from build123d import *

# Parameters (mm, degrees)
SKETCH2_R           = 1.5
BOSS_EXTRUDE2_DEPTH = 3


with BuildPart() as part:
    # Sketch2 → Boss-Extrude2 (new body)
    with BuildSketch(Plane.XY):
        with BuildLine():
            Line((33.856406461, -4.911436862), (20, -2.911436862))
            Line((20, -2.911436862), (8.072676136, 9.818872958))
            ThreePointArc((8.072676136, 9.818872958), (-5.173839679, 11.745880003), (-12.077884766, 0.277763382))
            ThreePointArc((-12.077884766, 0.277763382), (-13.37688471, -0.097129684), (-14.542044827, -0.782948586))
            ThreePointArc((-14.542044827, -0.782948586), (-14.504838322, -1.090725234), (-14.461118588, -1.3976444))
            ThreePointArc((-14.461118588, -1.3976444), (-13.158157346, -1.758528961), (-11.806390286, -1.78444193))
            ThreePointArc((-11.806390286, -1.78444193), (-11.67804324, -2.310249297), (-11.526291359, -2.829785359))
            ThreePointArc((-11.526291359, -2.829785359), (-12.683999488, -3.528110178), (-13.631954743, -4.492125996))
            ThreePointArc((-13.631954743, -4.492125996), (-13.516357561, -4.779785658), (-13.394691015, -5.064931306))
            ThreePointArc((-13.394691015, -5.064931306), (-12.042723303, -5.076287839), (-10.73030982, -4.751454786))
            ThreePointArc((-10.73030982, -4.751454786), (-10.470247132, -5.226127042), (-10.189200244, -5.688684064))
            ThreePointArc((-10.189200244, -5.688684064), (-11.126720661, -6.662850955), (-11.792869471, -7.839367605))
            ThreePointArc((-11.792869471, -7.839367605), (-11.606759368, -8.087306749), (-11.415437385, -8.331246676))
            ThreePointArc((-11.415437385, -8.331246676), (-10.106597569, -7.992301252), (-8.922976471, -7.338859012))
            ThreePointArc((-8.922976471, -7.338859012), (-8.548920985, -7.730048027), (-8.15773197, -8.104103513))
            ThreePointArc((-8.15773197, -8.104103513), (-8.81117421, -9.287724611), (-9.150119633, -10.596564427))
            ThreePointArc((-9.150119633, -10.596564427), (-8.906179706, -10.787886411), (-8.658240563, -10.973996513))
            ThreePointArc((-8.658240563, -10.973996513), (-7.481723913, -10.307847704), (-6.507557022, -9.370327286))
            ThreePointArc((-6.507557022, -9.370327286), (-6.045, -9.651374174), (-5.570327744, -9.911436862))
            ThreePointArc((-5.570327744, -9.911436862), (-5.895160797, -11.223850345), (-5.883804264, -12.575818057))
            ThreePointArc((-5.883804264, -12.575818057), (-5.598658616, -12.697484603), (-5.310998954, -12.813081785))
            ThreePointArc((-5.310998954, -12.813081785), (-4.346983136, -11.86512653), (-3.648658316, -10.707418401))
            ThreePointArc((-3.648658316, -10.707418401), (-3.129122255, -10.859170282), (-2.603314888, -10.987517329))
            ThreePointArc((-2.603314888, -10.987517329), (-2.577401919, -12.339284388), (-2.216517358, -13.64224563))
            ThreePointArc((-2.216517358, -13.64224563), (-1.909598192, -13.685965364), (-1.601821544, -13.723171869))
            ThreePointArc((-1.601821544, -13.723171869), (-0.916002642, -12.558011752), (-0.541109576, -11.259011808))
            ThreePointArc((-0.541109576, -11.259011808), (0, -11.271127042), (0.541109576, -11.259011808))
            ThreePointArc((0.541109576, -11.259011808), (0.916002642, -12.558011752), (1.601821544, -13.723171869))
            ThreePointArc((1.601821544, -13.723171869), (1.909598192, -13.685965364), (2.216517358, -13.64224563))
            ThreePointArc((2.216517358, -13.64224563), (2.577401919, -12.339284388), (2.603314888, -10.987517329))
            ThreePointArc((2.603314888, -10.987517329), (3.129122255, -10.859170282), (3.648658316, -10.707418401))
            ThreePointArc((3.648658316, -10.707418401), (4.346983136, -11.86512653), (5.310998954, -12.813081785))
            ThreePointArc((5.310998954, -12.813081785), (5.598658616, -12.697484603), (5.883804264, -12.575818057))
            ThreePointArc((5.883804264, -12.575818057), (5.895160797, -11.223850345), (5.570327744, -9.911436862))
            ThreePointArc((5.570327744, -9.911436862), (6.876145849, -9.125307162), (8.072676136, -8.181127042))
            Line((8.072676136, -8.181127042), (16, -11.911436862))
            Line((16, -11.911436862), (36, -11.911436862))
            Line((36, -11.911436862), (40, -13.911436862))
            ThreePointArc((40, -13.911436862), (43.70240259, -12.65581862), (42.40824957, -8.966708962))
            Line((42.40824957, -8.966708962), (33.856406461, -4.911436862))
        make_face()
        with Locations((41.229904242, -11.451628378)):
            Circle(SKETCH2_R, mode=Mode.SUBTRACT)
        with Locations((0, 0.818872958)):
            Circle(SKETCH2_R, mode=Mode.SUBTRACT)
    extrude(amount=BOSS_EXTRUDE2_DEPTH)


solid = part.part
Work out the finished part from the listing and answer in its coordinate system (mm). A direction names the side the tool comes from. Give positions to 0.01 mm unless a question says otherwise; leave off trailing zeros. Loops run counter-clockwise (first coordinate to the right, second up) from the corner with the lowest first, then second, coordinate; pieces in that order, holes last. Notation, with made-up numbers: (-3, 15.5) -> (38, 15.5) arc R20 ccw to (38, 19.5) -> close; hole circle Ø7 at (88.25, 1). An arc over 180 degrees is marked (long way). Use a Markdown table: item, result. Add a question column.
1. Section C-C on x = 38 is taken. Determine the outline of the cut face in (y, z), and give its area (3 significant figures).
2. A flat-ended cylindrical pin translates along its axis: pin 1 Ø2.5 at (x, y) = (0, 0.82) entering from +Z. Find the tip coordinate at first contact, or state that the pin passes through.
3. Section D-D on y = 3.75 is taken. Determine the outline of the cut face in (x, z), and give its area (3 significant figures).
4. Find the intervals of material crossed by probe 1 along Y at (x, z) = (0, 2.1); probe 2 along X at (y, z) = (-10.5, 0.95); probe 3 along X at (y, z) = (-12, 2.6), in increasing order.
5. Section A-A on x = 0 is taken. Determine the outline of the cut face in (y, z).
6. Section B-B on z = 2.4 is taken. State how many separate pieces and enclosed holes the cut face has, and give its area (3 significant figures).
7. Determine the mould class of faces 4 (the flat face through (8, -3, 0)), 5 (the cylindrical face through (-4.99, 11.83, 1.48)), 6 (the cylindrical face through (-4.36, -11.88, 1.48)) for opening direction X: released by +X, released by -X, zero draft, split by the parting line, or undercut.
8. For faces 1 (the cylindrical face through (-0.01, -11.27, 1.48)), 2 (the cylindrical face through (2.575, -12.358, 1.479)), 3 (the flat face through (38.192, -6.967, 1.479)), determine the directions among +Z, -Z, +X, -X, +Y, -Y from which every point of the face is accessible in a straight line to the end or side of a thin tool.
Results below:
| question | item | result |
|---|---|---|
| 1 | outline | (-12.91, 0) -> (-6.88, 0) -> (-6.88, 3) -> (-12.91, 3) -> close |
| 1 | area | 18.1 mm^2 |
| 2 | pin 1 | passes through |
| 3 | outline | (-11.73, 0) -> (13.76, 0) -> (13.76, 3) -> (-11.73, 3) -> close |
| 3 | area | 76.5 mm^2 |
| 4 | probe 1 | y = -11.27 to -0.68, 2.32 to 12.91 |
| 4 | probe 2 | x = -9.14 to -7.76, -5.76 to 5.76, 13 to 40.07, 42.39 to 43.81 |
| 4 | probe 3 | x = -5.93 to -4.46, -2.62 to -0.71, 0.71 to 2.62, 4.46 to 5.93, 36.18 to 39.83, 42.63 to 43.92 |
| 5 | outline | (-11.27, 0) -> (-0.68, 0) -> (-0.68, 3) -> (-11.27, 3) -> close; (2.32, 0) -> (12.91, 0) -> (12.91, 3) -> (2.32, 3) -> close |
| 6 | separate pieces | 1 |
| 6 | enclosed holes | 2 |
| 6 | area | 764 mm^2 |
| 7 | face 4 | zero draft |
| 7 | face 5 | split by the parting line |
| 7 | face 6 | undercut |
| 8 | face 1 | +Z, -Z, -Y |
| 8 | face 2 | +Z, -Z |
| 8 | face 3 | +Z, -Z, +X, +Y |
